```python
from build123d import *

# Parameters (mm, degrees)
CROQUIS1_R               = 3
SALIENTE_EXTRUIR1_DEPTH  = 1
CROQUIS2_R               = 3.5
CROQUIS2_R_2             = 3
SALIENTE_EXTRUIR2_DEPTH  = 7
SALIENTE_EXTRUIR3_START  = 1
CROQUIS3_R               = 4
CROQUIS3_R_2             = 3
SALIENTE_EXTRUIR3_DEPTH  = 1
CORTAR_EXTRUIR3_DEPTH    = 0.2
REDONDEO4_R              = 1.5
REDONDEO4_OF_SIMETR_A4_R = 1.5


with BuildPart() as part:
    # Croquis1 → Saliente-Extruir1 (new body)
    with BuildSketch(Plane(origin=(0, 0, 0), x_dir=(1, 0, 0), z_dir=(0, 1, 0))):
        with BuildLine():
            Line((-50.264827345, 5.804943896), (-54.04727716, 15.061999227))
            ThreePointArc((-54.04727716, 15.061999227), (-59.890614713, 22.75333698), (-58.675804825, 13.17077432))
            Line((-58.675804825, 13.17077432), (-54.893355011, 3.913718989))
            ThreePointArc((-54.893355011, 3.913718989), (-49.050017457, -3.777618763), (-50.264827345, 5.804943896))
        make_face()
        with Locations(Location((-57.999389806, 18.124809314, 0), (0, 0, 270))):
            Circle(CROQUIS1_R, mode=Mode.SUBTRACT)
        with Locations(Location((-50.941242364, 0.850908902, 0), (0, 0, 270))):
            Circle(CROQUIS1_R, mode=Mode.SUBTRACT)
    extrude(amount=SALIENTE_EXTRUIR1_DEPTH)

    # Croquis2 → Saliente-Extruir2 (add)
    # profile 1 of 2: a face of its own
    with BuildSketch(Plane(origin=(0, 1, 0), x_dir=(1, 0, 0), z_dir=(0, 1, 0))):
        with Locations(Location((-50.941242364, 0.850908902, 0), (0, 0, 270))):
            Circle(CROQUIS2_R)
        with Locations(Location((-50.941242364, 0.850908902, 0), (0, 0, 270))):
            Circle(CROQUIS2_R_2, mode=Mode.SUBTRACT)
    # profile 2 of 2: a face of its own
    with BuildSketch(Plane(origin=(0, 1, 0), x_dir=(1, 0, 0), z_dir=(0, 1, 0))):
        with Locations(Location((-57.999389806, 18.124809314, 0), (0, 0, 270))):
            Circle(CROQUIS2_R)
        with Locations(Location((-57.999389806, 18.124809314, 0), (0, 0, 270))):
            Circle(CROQUIS2_R_2, mode=Mode.SUBTRACT)
    extrude(amount=SALIENTE_EXTRUIR2_DEPTH)

    # Croquis3 → Saliente-Extruir3 (add)
    with BuildSketch(Plane.XZ.offset(SALIENTE_EXTRUIR3_START)):
        with Locations(Location((-50.941242364, -0.850908902, 0), (0, 0, 90))):
            Circle(CROQUIS3_R)
        with Locations(Location((-50.941242364, -0.850908902, 0), (0, 0, 270))):
            Circle(CROQUIS3_R_2, mode=Mode.SUBTRACT)
    extrude(amount=-SALIENTE_EXTRUIR3_DEPTH)

    # Croquis4 → Cortar-Extruir3 (cut)
    with BuildSketch(Plane.XZ):
        with BuildLine():
            Line((-55.03045688, -6.89304724), (-53.64189858, -7.460414712))
            Line((-53.64189858, -7.460414712), (-53.074531108, -6.071856412))
            ThreePointArc((-53.074531108, -6.071856412), (-54.222568183, -6.077366335), (-55.03045688, -6.89304724))
        make_face()
        with BuildLine():
            Line((-53.074531108, -6.071856412), (-53.64189858, -7.460414712))
            Line((-53.64189858, -7.460414712), (-52.253340281, -8.027782184))
            ThreePointArc((-52.253340281, -8.027782184), (-52.258850203, -6.879745109), (-53.074531108, -6.071856412))
        make_face()
        Polygon((-52.253340281, -8.027782184), (-53.64189858, -7.460414712), (-55.29873359, -11.515303505), (-53.91017529, -12.082670977), align=None)
        Polygon((-55.29873359, -11.515303505), (-53.64189858, -7.460414712), (-55.03045688, -6.89304724), (-56.68729189, -10.947936033), align=None)
        with BuildLine():
            Line((-53.91017529, -12.082670977), (-55.29873359, -11.515303505))
            Line((-55.29873359, -11.515303505), (-55.866101062, -12.903861804))
            ThreePointArc((-55.866101062, -12.903861804), (-54.718063987, -12.898351882), (-53.91017529, -12.082670977))
        make_face()
        with BuildLine():
            Line((-55.866101062, -12.903861804), (-55.29873359, -11.515303505))
            Line((-55.29873359, -11.515303505), (-56.68729189, -10.947936033))
            ThreePointArc((-56.68729189, -10.947936033), (-56.681781967, -12.095973108), (-55.866101062, -12.903861804))
        make_face()
    cortar_extruir3 = extrude(amount=-CORTAR_EXTRUIR3_DEPTH, mode=Mode.SUBTRACT)

    # Redondeo4
    # the kernel refuses this fillet: 1.5 mm, written as the material it adds along each edge
    with BuildSketch(Plane(origin=(-55.29873359, 0.2, -11.515303505), x_dir=(0.9257055331084191, 0, -0.3782449814240206), z_dir=(0.3782449814240206, 0, 0.9257055331084191))) as redondeo4_piece_1:
        with BuildLine():
            CenterArc((0.751668523, -1.5), REDONDEO4_R, 60.073565133, 29.926434867)
            Line((0.751668523, 0), (0.751668523, 0.03))
            Line((0.751668523, 0.03), (1.5, 0.03))
            Line((1.5, 0.03), (1.53, 0))
            ThreePointArc((1.53, 0), (1.53, -0.1), (1.51496663, -0.174))
            Line((1.51496663, -0.174), (1.5, -0.2))
        make_face()
    revolve(axis=Axis((-55.29873359, 0.2, -11.515303505), (0, 1, 0)), revolution_arc=180)
    with BuildSketch(Plane(origin=(-53.91017529, 0.2, -12.082670977), x_dir=(0, -1, 0), z_dir=(0.37824498142401725, 0, 0.9257055331084204)), Plane(origin=(-55.03045688, 0.2, -6.89304724), x_dir=(0, -1, 0), z_dir=(-0.3782449814240187, 0, -0.9257055331084199))) as redondeo4_piece_2:
        with BuildLine():
            CenterArc((1.5, -0.748331477), REDONDEO4_R, 150.073565133, 29.926434867)
            Line((0, -0.748331477), (-0.03, -0.748331477))
            Line((-0.03, -0.748331477), (-0.03, 0))
            Line((-0.03, 0), (0, 0.03))
            ThreePointArc((0, 0.03), (0.1, 0.03), (0.174, 0.01496663))
            Line((0.174, 0.01496663), (0.2, 0))
        make_face()
    extrude(amount=4.380322519)
    with BuildSketch(Plane(origin=(-53.64189858, 0.2, -7.460414712), x_dir=(0.9257055331084226, 0, -0.378244981424012), z_dir=(-0.378244981424012, 0, -0.9257055331084226))) as redondeo4_piece_3:
        with BuildLine():
            CenterArc((0.751668523, 1.5), REDONDEO4_R, 270, 29.926434867)
            Line((0.751668523, 0), (0.751668523, -0.03))
            Line((0.751668523, -0.03), (1.5, -0.03))
            Line((1.5, -0.03), (1.53, 0))
            ThreePointArc((1.53, 0), (1.53, 0.1), (1.51496663, 0.174))
            Line((1.51496663, 0.174), (1.5, 0.2))
        make_face()
    revolve(axis=Axis((-53.64189858, 0.2, -7.460414712), (0, -1, 0)), revolution_arc=180)

    # Simetría4: Cortar-Extruir3 across plane
    add(cortar_extruir3.mirror(Plane(origin=(0, 0.5, 0), x_dir=(0, 0, 1), z_dir=(0, -1, 0))), mode=Mode.SUBTRACT)

    # Redondeo4 of Simetría4
    # the kernel refuses this fillet: 1.5 mm, written as the material it adds along each edge
    with BuildSketch(Plane(origin=(-55.29873359, 0.8, -11.515303505), x_dir=(0.9257055331084191, 0, -0.3782449814240206), z_dir=(0.3782449814240206, 0, 0.9257055331084191))) as redondeo4_of_simetr_a4_piece_1:
        with BuildLine():
            CenterArc((0.751668523, 1.5), REDONDEO4_OF_SIMETR_A4_R, 270, 29.926434867)
            Line((0.751668523, 0), (0.751668523, -0.03))
            Line((0.751668523, -0.03), (1.5, -0.03))
            Line((1.5, -0.03), (1.53, 0))
            ThreePointArc((1.53, 0), (1.53, 0.1), (1.51496663, 0.174))
            Line((1.51496663, 0.174), (1.5, 0.2))
        make_face()
    revolve(axis=Axis((-55.29873359, 0.8, -11.515303505), (0, 1, 0)), revolution_arc=180)
    with BuildSketch(Plane(origin=(-53.91017529, 0.8, -12.082670977), x_dir=(0, 1, 0), z_dir=(0.37824498142401725, 0, 0.9257055331084204)), Plane(origin=(-55.03045688, 0.8, -6.89304724), x_dir=(0, 1, 0), z_dir=(-0.3782449814240187, 0, -0.9257055331084199))) as redondeo4_of_simetr_a4_piece_2:
        with BuildLine():
            CenterArc((1.5, 0.748331477), REDONDEO4_OF_SIMETR_A4_R, 180, 29.926434867)
            Line((0, 0.748331477), (-0.03, 0.748331477))
            Line((-0.03, 0.748331477), (-0.03, 0))
            Line((-0.03, 0), (0, -0.03))
            ThreePointArc((0, -0.03), (0.1, -0.03), (0.174, -0.01496663))
            Line((0.174, -0.01496663), (0.2, 0))
        make_face()
    extrude(amount=4.380322519)
    with BuildSketch(Plane(origin=(-53.64189858, 0.8, -7.460414712), x_dir=(0.9257055331084226, 0, -0.378244981424012), z_dir=(-0.378244981424012, 0, -0.9257055331084226))) as redondeo4_of_simetr_a4_piece_3:
        with BuildLine():
            CenterArc((0.751668523, -1.5), REDONDEO4_OF_SIMETR_A4_R, 60.073565133, 29.926434867)
            Line((0.751668523, 0), (0.751668523, 0.03))
            Line((0.751668523, 0.03), (1.5, 0.03))
            Line((1.5, 0.03), (1.53, 0))
            ThreePointArc((1.53, 0), (1.53, -0.1), (1.51496663, -0.174))
            Line((1.51496663, -0.174), (1.5, -0.2))
        make_face()
    revolve(axis=Axis((-53.64189858, 0.8, -7.460414712), (0, -1, 0)), revolution_arc=180)


solid = part.part
```
Build history of the part. All positions in model axes, mm. A direction names the side the tool comes from. Give positions to 0.01 mm unless a question says otherwise; leave off trailing zeros. Order: outer loops, then holes, each group sorted by start corner. A loop starts at its lowest first (then second) coordinate and runs counter-clockwise, first axis right, second up. Notation, with made-up numbers: M 55,17.5 L 68,17.5 A29 ccw 68,41.5 Z; hole C -9.5,17.5 d4. An arc over 180 degrees is marked long. Write item = value, one per line. Start each with the question number.
(1) Pin check, flat tips, straight feed: pin 1 Ø8 at (x, z) = (-50.5, -13.5) entering from -Y; pin 2 Ø1.6 at (x, z) = (-54.5, -8.5) entering from +Y; pin 3 Ø1.5 at (y, z) = (5, -15.5) entering from +X. Stop position of each tip, or through.
(2) Probe L1, parallel to X at y = 7.5, z = -3; L2, parallel to X at y = 6.5, z = -1.75; L3, parallel to Y at x = -55.75, z = -13. List the from-to ranges inside material, lowest first. Write a range as [from, to].
(3) Which spindle directions (+Z, -Z, +X, -X, +Y, -Y) get a long thin tool onto all of the face, cutting with end or side? Do faces 4 (the flat face through (-54, 0.2, -9)), 5 (the flat face through (-57, 8, -15)), 6 (the cylindrical face through (-61.1, 4.5, -16.5)), 7 (the cylindrical face through (-60.928, 3.944, -18.775)), 8 (the flat face through (-56.811, 0.493, -8.607)). Say none if no direction does.
(4) Slice it at D-D on y = -0.5. Write the cut outline in (x, z).
(5) Slice it at C-C on y = 5. Write the cut outline in (x, z), plus the area to 3 significant figures.
(6) Slice it at A-A on x = -51.5. Write the cut outline in (y, z).
(7) Slice it at B-B on z = -3. Write the cut outline in (x, y).
(8) Two-plate mould, pull along Z, no slides. Class faces 1 (the cylindrical face through (-53.423, 0.148, -9.949)), 2 (the flat face through (-57, 0, -12)), 3 (the cylindrical face through (-47.036, -0.507, -1.718)): released by +Z, released by -Z, zero draft, split by the parting line, or undercut.
Responses:
q1.pin_1 = 0
q1.pin_2 = 0.87
q1.pin_3 = -55.04
q2.L1 = [-53.7, -53.03], [-48.85, -48.18]
q2.L2 = [-54.32, -53.8], [-48.08, -47.56]
q2.L3 = [0, 1]
q3.face_4 = -Y
q3.face_5 = +Z, -Z, +X, -X, +Y
q3.face_6 = +Y
q3.face_7 = +Y, -Y
q3.face_8 = -X, +Y, -Y
q4.outline = C -50.94,-0.85 d8; hole C -50.94,-0.85 d6
q5.outline = C -58,-18.12 d7; C -50.94,-0.85 d7; hole C -58,-18.12 d6; hole C -50.94,-0.85 d6
q5.area = 20.4 mm2
q6.outline = M -1,-4.81 L 0,-4.81 L 0,-8.83 L 1,-8.83 L 1,-4.31 L 8,-4.31 L 8,-3.8 L -1,-3.8 Z; M -1,2.1 L 8,2.1 L 8,2.6 L 1,2.6 L 1,4.12 L 0,4.12 L 0,3.11 L -1,3.11 Z
q7.outline = M -55.46,0 L -54.31,0 L -54.31,-1 L -53.03,-1 L -53.03,8 L -53.7,8 L -53.7,1 L -55.46,1 Z; M -48.85,-1 L -47.57,-1 L -47.57,0 L -46.43,0 L -46.43,1 L -48.18,1 L -48.18,8 L -48.85,8 Z
q8.face_1 = undercut
q8.face_2 = zero draft
q8.face_3 = split by the parting line
